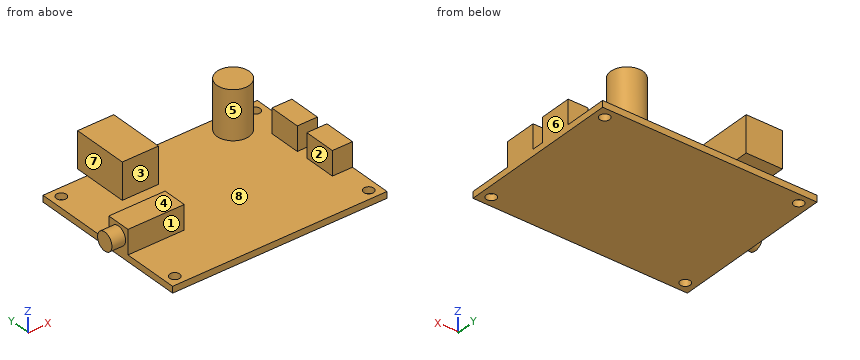
```python
from build123d import *

# Parameters (mm, degrees)
ESQUISSE1_W        = 53.34
ESQUISSE1_H        = 40.64
ESQUISSE1_R        = 1.25
BOSS_EXTRU_1_DEPTH = 1.6
ESQUISSE2_W        = 14
ESQUISSE2_H        = 6
ESQUISSE2_W_2      = 5
ESQUISSE2_H_2      = 8
BOSS_EXTRU_2_DEPTH = 6
ESQUISSE3_R        = 2.25
BOSS_EXTRU_3_DEPTH = 3.4
ESQUISSE4_W        = 9
ESQUISSE4_H        = 14
BOSS_EXTRU_4_DEPTH = 9
ESQUISSE5_R        = 4
BOSS_EXTRU_5_DEPTH = 12


with BuildPart() as part:
    # Esquisse1 → Boss.-Extru.1 (new body)
    with BuildSketch(Plane.XY):
        Rectangle(ESQUISSE1_W, ESQUISSE1_H)
        with Locations((-24.13, 17.78)):
            Circle(ESQUISSE1_R, mode=Mode.SUBTRACT)
        with Locations((24.13, -17.78)):
            Circle(ESQUISSE1_R, mode=Mode.SUBTRACT)
        with Locations((24.13, 17.78)):
            Circle(ESQUISSE1_R, mode=Mode.SUBTRACT)
        with Locations((-24.13, -17.78)):
            Circle(ESQUISSE1_R, mode=Mode.SUBTRACT)
    extrude(amount=BOSS_EXTRU_1_DEPTH)

    # Esquisse2 → Boss.-Extru.2 (add)
    with BuildSketch(Plane.XY.offset(1.6)):
        with Locations((-19.67, -3.32)):
            Rectangle(ESQUISSE2_W, ESQUISSE2_H)
        with Locations((24.17, 5.5)):
            Rectangle(ESQUISSE2_W_2, ESQUISSE2_H_2)
        with Locations((24.17, -5.5)):
            Rectangle(ESQUISSE2_W_2, ESQUISSE2_H_2)
    extrude(amount=BOSS_EXTRU_2_DEPTH)

    # Esquisse3 → Boss.-Extru.3 (add)
    with BuildSketch(Plane.ZY.offset(26.67)):
        with Locations(Location((4.6, -3.32, 0), (0, 0, 270))):
            Circle(ESQUISSE3_R)
    extrude(amount=BOSS_EXTRU_3_DEPTH)

    # Esquisse4 → Boss.-Extru.4 (add)
    with BuildSketch(Plane.XY.offset(1.6)):
        with Locations((-11.17, 16.32)):
            Rectangle(ESQUISSE4_W, ESQUISSE4_H)
    extrude(amount=BOSS_EXTRU_4_DEPTH)

    # Esquisse5 → Boss.-Extru.5 (add)
    with BuildSketch(Plane.XY.offset(1.6)):
        with Locations((16.67, 15.32)):
            Circle(ESQUISSE5_R)
    extrude(amount=BOSS_EXTRU_5_DEPTH)


solid = part.part
```
Verification items for the finished model (mm, model axes). Face numbers are marked on the shaded views. A direction names the side the tool comes from. Give positions to 0.01 mm unless a question says otherwise; leave off trailing zeros. Loops run counter-clockwise (first coordinate to the right, second up) from the corner with the lowest first, then second, coordinate; pieces in that order, holes last. Notation, with made-up numbers: M 14.25,77 L 30.25,77 A25 ccw 30.25,96 Z; hole C 58,68.25 d11. An arc over 180 degrees is marked long. Return JSON: item names as keys, results as strings.
1) Gauge pin test, flat ends, axial feed: P1, Ø8, axis at x = 6.5, y = 8.5, coming from the +Z side; P2, Ø8, axis at x = -11.5, y = -4, coming from the +Z side; P3, Ø0.9, axis at x = -9, y = 22, coming from the -Z side; P4, Ø2, axis at x = 24.13, y = -17.78, coming from the +Z side. Record the tip position at first contact, or that the pin passes through.
Findings:
{"P1": "stops at z = 1.6", "P2": "stops at z = 7.6", "P3": "stops at z = 1.6", "P4": "passes through"}
2) Section check D-D, the plane x = -9. Enter the section's corners in (y, z), and give its area (3 significant figures).
Findings:
{"outline": "M -20.32,0 L 20.32,0 L 20.32,1.6 L 23.32,1.6 L 23.32,10.6 L 9.32,10.6 L 9.32,1.6 L -20.32,1.6 Z", "area": "191 mm2"}
3) Material ranges on L1, parallel to Y at x = -24.13, z = 0.95; L2, parallel to X at y = 5, z = 5.25; L3, parallel to Z at x = -8, y = -14, recorded low to high. Write a range as [from, to].
Findings:
{"L1": "y = [-20.32, -19.03], [-16.53, 16.53], [19.03, 20.32]", "L2": "x = [21.67, 26.67]", "L3": "z = [0, 1.6]"}
4) Mould release check, pull along X, two halves, no side actions. Record for the marked faces 5, 6, 7 and 8: released by +X, released by -X, zero draft, split by the parting line, or undercut.
Findings:
{"face 5": "undercut", "face 6": "released by +X", "face 7": "released by -X", "face 8": "undercut"}
5) Section check A-A, the plane x = -24.13. Enter the section's corners in (y, z).
Findings:
{"outline": "M -20.32,0 L -19.03,0 L -19.03,1.6 L -20.32,1.6 Z; M -16.53,0 L 16.53,0 L 16.53,1.6 L -0.32,1.6 L -0.32,7.6 L -6.32,7.6 L -6.32,1.6 L -16.53,1.6 Z; M 19.03,0 L 20.32,0 L 20.32,1.6 L 19.03,1.6 Z"}
6) Section check C-C, the plane y = -17.78. Enter the section's corners in (x, z), and give its area (3 significant figures).
Findings:
{"outline": "M -26.67,0 L -25.38,0 L -25.38,1.6 L -26.67,1.6 Z; M -22.88,0 L 22.88,0 L 22.88,1.6 L -22.88,1.6 Z; M 25.38,0 L 26.67,0 L 26.67,1.6 L 25.38,1.6 Z", "area": "77.3 mm2"}
7) Tool access check on the marked faces 1, 2, 3 and 4. Record the directions out of +Z, -Z, +X, -X, +Y, -Y that give a thin tool (end or side, any length) a straight path to the whole face; none if there is none.
Findings:
{"face 1": "+Z, -X, -Y", "face 2": "+Z, +Y, -Y", "face 3": "+Z, -X", "face 4": "+Z, +X, -X, -Y"}
8) Section check B-B, the plane z = 4.6. Enter the section's corners in (x, y).
Findings:
{"outline": "M -30.07,-5.57 L -26.67,-5.57 L -26.67,-6.32 L -12.67,-6.32 L -12.67,-0.32 L -26.67,-0.32 L -26.67,-1.07 L -30.07,-1.07 Z; M -15.67,9.32 L -6.67,9.32 L -6.67,23.32 L -15.67,23.32 Z; C 16.67,15.32 d8; M 21.67,-9.5 L 26.67,-9.5 L 26.67,-1.5 L 21.67,-1.5 Z; M 21.67,1.5 L 26.67,1.5 L 26.67,9.5 L 21.67,9.5 Z"}
